Verification items for the finished model (mm, model axes). A direction names the side the tool comes from. Round coordinates to 2 decimals unless told otherwise and drop trailing zeros. Order: outer loops, then holes, each group sorted by start corner. A loop starts at its lowest first (then second) coordinate and runs counter-clockwise, first axis right, second up. Notation, with made-up numbers: (-4, -22) -> (35, -22) arc R15 ccw to (35, 2) -> close; hole circle Ø3 at (22, 54.25). An arc over 180 degrees is marked (long way). Return JSON: item names as keys, results as strings. Group by question number.
1) Scan lines: L1, parallel to Z at x = 2.65, y = -13.5; L2, parallel to Y at x = 4, z = 13.5; L3, parallel to Z at x = 2.45, y = -11.5. Record each from-to range of solid material in increasing order.
2) Section check A-A on y = -3. Enter the section's corners in (x, z), plus the area to 3 significant figures.
3) Draft check along Y on faces 5 (the flat face through (2.535, 2.799, -1.647)), 6 (the cylindrical face through (2.5, 12.9, -5.7)). Enter one of: pulls with the +Y half, pulls with the -Y half, needs draft (parallel to the pull), parting line crosses it, or undercut.
4) Section check B-B on y = 0.5. Enter the section's corners in (x, z), plus the area to 3 significant figures.
5) Section check D-D on y = -7. Enter the section's corners in (x, z), plus the area to 3 significant figures.
6) Tool access check on faces 1 (the cylindrical face through (2.46, -1.03, -12.33)), 2 (the cylindrical face through (2.46, 10.36, 9.6)), 3 (the cylindrical face through (2.46, -4.54, 13.42)), 4 (the cylindrical face through (2.46, -2.37, 13.92)). Record the directions out of +Z, -Z, +X, -X, +Y, -Y that give a thin tool (end or side, any length) a straight path to the whole face; none if there is none.
7) Section check C-C on y = 8. Enter the section's corners in (x, z).
8) Depth check by flat-ended pin: pin 1 (12 mm diameter, centred on y = -12, z = 3.5, fed in from -X); pin 2 (3 mm diameter, centred on x = 4, z = -3.5, fed in from -Y); pin 3 (1 mm diameter, centred on x = 1.5, z = 9, fed in from +Y); pin 4 (1 mm diameter, centred on x = 2, z = -10, fed in from +Y). Enter the tip coordinate at first touch or a pass-through.
```python
from build123d import *

# Parameters (mm, degrees)
BASPROSKE_W     = 5
BASPROSKE_H     = 15.75
TOOTHCUT_DEPTH  = 23.828162432
TEETHCUTS_COUNT = 19
TEETHCUTS_ANGLE = 341.052631579
BORE_DEPTH      = 50.0000508


with BuildPart() as part:
    # BasProSke → Base-Revolve (revolve)
    with BuildSketch(Plane(origin=(0, 0, 0), x_dir=(1, 0, 0), z_dir=(0, 1, 0)), mode=Mode.PRIVATE) as base_revolve_sk:
        with Locations((2.5, 7.875)):
            Rectangle(BASPROSKE_W, BASPROSKE_H)
    revolve(base_revolve_sk.sketch.rotate(Axis((-10, 0, 0), (1, 0, 0)), 180), axis=Axis((-10, 0, 0), (1, 0, 0)))

    # TooCutSke → ToothCut (cut, through all)
    with BuildSketch(Plane(origin=(0, 0, 0), x_dir=(0, 0, -1), z_dir=(1, 0, 0))):
        with BuildLine():
            ThreePointArc((0.751505376, 12.351158475), (0, 12.374), (-0.751505376, 12.351158475))
            ThreePointArc((-0.751505376, 12.351158475), (-1.227741339, 14.103349268), (-2.230855439, 15.616866817))
            ThreePointArc((-2.230855439, 15.616866817), (0, 15.7754), (2.230855439, 15.616866817))
            ThreePointArc((2.230855439, 15.616866817), (1.227741339, 14.103349268), (0.751505376, 12.351158475))
        make_face()
    toothcut = extrude(amount=TOOTHCUT_DEPTH, mode=Mode.SUBTRACT)

    # TeethCuts: ToothCut ×19 about axis
    teethcuts_axis = Axis((-10, 0, 0), (1, 0, 0))
    for i in range(1, TEETHCUTS_COUNT):
        add(toothcut.rotate(teethcuts_axis, i * TEETHCUTS_ANGLE / (TEETHCUTS_COUNT - 1)), mode=Mode.SUBTRACT)

    # BorSke → Bore (cut, symmetric)
    with BuildSketch(Plane(origin=(0, 0, 0), x_dir=(0, 0, -1), z_dir=(1, 0, 0))):
        Polygon((0, 3.75), (-3.247595264, 1.875), (-3.247595264, -1.875), (0, -3.75), (3.247595264, -1.875), (3.247595264, 1.875), align=None)
    extrude(amount=BORE_DEPTH, both=True, mode=Mode.SUBTRACT)


solid = part.part
```
Check result:
{
 "1": {"L1": "-5.65 to -3.4, -1.24 to 1.24, 3.4 to 5.65", "L2": "-4.54 to -2.16, -0.13 to 2.34, 4.76 to 6.75", "L3": "-9.87 to -7.41, -5.32 to 5.32, 7.41 to 9.87"},
 "2": {"outline": "(0, -14.84) -> (5, -14.84) -> (5, -1.3) -> (0, -1.3) -> close; (0, 1.3) -> (5, 1.3) -> (5, 14.84) -> (0, 14.84) -> close", "area": "135 mm^2"},
 "3": {"face 5": "undercut", "face 6": "pulls with the +Y half"},
 "4": {"outline": "(0, -15.11) -> (5, -15.11) -> (5, -3.25) -> (0, -3.25) -> close; (0, 3.25) -> (5, 3.25) -> (5, 15.11) -> (0, 15.11) -> close", "area": "119 mm^2"},
 "5": {"outline": "(0, -12.6) -> (5, -12.6) -> (5, 12.6) -> (0, 12.6) -> close", "area": "126 mm^2"},
 "6": {"face 1": "-Z, +X, -X", "face 2": "+X, -X, +Y", "face 3": "+X, -X", "face 4": "+Z, +X, -X"},
 "7": {"outline": "(0, -10.57) -> (5, -10.57) -> (5, 10.57) -> (0, 10.57) -> close"},
 "8": {"pin 1": "x = 0", "pin 2": "y = -15.02", "pin 3": "y = 10.3", "pin 4": "y = 10.74"}
}
